```python
from build123d import *

# Parameters (mm, degrees)
F0_W     = 64.236599952
F0_H     = 76.123803854
F1_DEPTH = 18
F2_W     = 64.236599952
F2_H     = 54.1637830138
F3_DEPTH = 76
F5_T     = -13
F4_R     = 12.5879419165
F6_DEPTH = 205.6


with BuildPart() as f1:
    # F0 (on Top) → F1 (new body)
    with BuildSketch(Plane.XY):
        with Locations((-4.2166989297, -5.8254562318)):
            Rectangle(F0_W, F0_H)
        with BuildLine():
            Line((-36.3349989057, -43.8873581588), (-36.3349989057, 32.2364456952))
            ThreePointArc((-36.3349989057, 32.2364456952), (-74.3969008327, -5.8254562318), (-36.3349989057, -43.8873581588))
        make_face()
    extrude(amount=F1_DEPTH)

    # F2 (on face) → F3 (join)
    with BuildSketch(Plane(origin=(0, 32.2364456952, 0), x_dir=(-1, 0, 0), z_dir=(0, 1, 0))):
        with Locations((4.2166989297, 45.0818915069)):
            Rectangle(F2_W, F2_H)
    extrude(amount=-F3_DEPTH)

    # F5
    f5_openings = [f1.faces().sort_by_distance(p)[0] for p in [
        (-4.216699, -5.763554, 72.163783),
    ]]
    offset(amount=F5_T, openings=f5_openings, kind=Kind.INTERSECTION)

    # F4 (on face) → F6 (cut)
    with BuildSketch(Plane.XZ.offset(43.7635543048)):
        with Locations((-7.7566844411, 36.2076386809)):
            Circle(F4_R)
    extrude(amount=-F6_DEPTH, mode=Mode.SUBTRACT)


solid = f1.part
```
Design review of the part built by this model. Coordinates are the model's own, in mm. A direction names the side the tool comes from. Give positions to 0.01 mm unless a question says otherwise; leave off trailing zeros. Order: outer loops, then holes, each group sorted by start corner. A loop starts at its lowest first (then second) coordinate and runs counter-clockwise, first axis right, second up. Notation, with made-up numbers: (-8.5, 9) - (43.5, 9) arc R26 ccw to (43.5, 29) - close; hole circle Ø8 at (54, 9). An arc over 180 degrees is marked (long way). Use a Markdown table: item, result. Add a question column.
(1) Add section C-C on z = 21. Give the boundary of the cut face in (x, y) (3 decimals), then the cut area to 3 significant figures.
(2) Machinability: for faces 1 (the face through (-4, -30.764, 50)), 2 (the face through (-36.335, -5, 45)), 3 (the face through (-24, -5, 0)), which of the approach directions +Z, -Z, +X, -X, +Y, -Y give a long, thin tool a straight path to every point of the face, cutting with its end or side? Answer none if there is none.
(3) Add section D-D on y = -6.5. Give the boundary of the cut face in (x, z) (3 decimals).
(4) Clearance check with flat-ended pins moving along their axes: P1, Ø22.5, axis at x = -7.76, z = 36.21, coming from the +Y side; P2, Ø6, axis at x = -59.5, y = -13.5, coming from the +Z side; P3, Ø16, axis at x = 0, z = 43.5, coming from the -Y side; P4, Ø2, axis at y = 8, z = 31.5, coming from the -X side (3 decimals). State where each tip first meets the part, or that it passes through.
(5) Add section A-A on z = 42.5. Give the boundary of the cut face in (x, y) (3 decimals), then the cut area to 3 significant figures.
(6) Wall thickness on probe 1 along X at (y, z) = (-22, 60) (3 decimals); probe 2 along Y at (x, z) = (-2.5, 57); probe 3 along Z at (x, y) = (-41.5, 28): over which ranges is each line inside the solid? List them lowest first. Write a range as [from, to].
(7) Mouldability with a two-part tool opening along Y and no side actions: class faces 4 (the face through (-10.49, 25.65, 23.92)), 5 (the face through (-23.335, -5, 42)), 6 (the face through (-4, 19.236, 50)), 7 (the face through (-4, -43.764, 51)) as +Y half, -Y half, draft (parallel to the pull), parting line (faces both ways), or undercut.
(8) Add section B-B on y = -35.5. Give the boundary of the cut face in (x, z) (3 decimals).
Report:
| question | item | result |
|---|---|---|
| 1 | outline | (-36.335, -43.764) - (27.902, -43.764) - (27.902, 32.236) - (-36.335, 32.236) - close; hole (-23.335, -30.764) - (14.902, -30.764) - (14.902, 19.236) - (-23.335, 19.236) - close |
| 1 | area | 2,970 mm² |
| 2 | face 1 | +Z |
| 2 | face 2 | +Z, -X, +Y, -Y |
| 2 | face 3 | -Z, +X, -X, +Y, -Y |
| 3 | outline | (-74.391, 0) - (27.902, 0) - (27.902, 72.164) - (14.902, 72.164) - (14.902, 13) - (-23.335, 13) - (-23.335, 72.164) - (-36.335, 72.164) - (-36.335, 18) - (-74.391, 18) - close |
| 4 | P1 | passes through |
| 4 | P2 | stops at z = 18 |
| 4 | P3 | stops at y = -43.76 |
| 4 | P4 | stops at x = -36.335 |
| 5 | outline | (-36.335, -43.764) - (-18.659, -43.764) - (-18.659, -30.764) - (-23.335, -30.764) - (-23.335, 19.236) - (-18.659, 19.236) - (-18.659, 32.236) - (-36.335, 32.236) - close; (3.146, -43.764) - (27.902, -43.764) - (27.902, 32.236) - (3.146, 32.236) - (3.146, 19.236) - (14.902, 19.236) - (14.902, -30.764) - (3.146, -30.764) - close |
| 5 | area | 2,400 mm² |
| 6 | probe 1 | x = [-36.335, -23.335], [14.902, 27.902] |
| 6 | probe 2 | y = [-43.76, -30.76], [19.24, 32.24] |
| 6 | probe 3 | z = [0, 18] |
| 7 | face 4 | draft |
| 7 | face 5 | undercut |
| 7 | face 6 | undercut |
| 7 | face 7 | -Y half |
| 8 | outline | (-60.17, 0) - (27.902, 0) - (27.902, 72.164) - (-36.335, 72.164) - (-36.335, 18) - (-60.17, 18) - close; hole circle Ø25.176 at (-7.757, 36.208) |
